CAD build for the part. Positions are in the model's coordinates, mm. Face numbers are marked on the shaded views. A direction names the side the tool comes from. Give positions to 0.01 mm unless a question says otherwise; leave off trailing zeros. Loops run counter-clockwise (first coordinate to the right, second up) from the corner with the lowest first, then second, coordinate; pieces in that order, holes last.
Autodesk Inventor part; units mm, degrees
ref_plane "YZ Plane" through (0, 0, 0) normal (1, 0, 0) x (0, 1, 0)
ref_plane "XZ Plane" through (0, 0, 0) normal (0, 1, 0) x (-1, 0, 0)
ref_plane "XY Plane" through (0, 0, 0) normal (0, 0, 1) x (1, 0, 0)
sketch "草图1" plane through (0, 0, 0) normal (0, 0, 1) x (1, 0, 0)
  circle A0 centre (0, 0) radius 4
  dimension "d0" = 8
extrude "拉伸1" add sketch "草图1" along normal blind 1
sketch "草图2" plane through (0, 0, 1) normal (0, 0, 1) x (1, 0, 0)
  line L0 (0, -2.8868) -> (-2.5, -1.4434)
  line L1 (-2.5, -1.4434) -> (-2.5, 1.4434)
  line L2 (-2.5, 1.4434) -> (0, 2.8868)
  line L3 (0, 2.8868) -> (2.5, 1.4434)
  line L4 (2.5, 1.4434) -> (2.5, -1.4434)
  line L5 (2.5, -1.4434) -> (0, -2.8868)
  point P0 (0, 0)
  point P1 (0, 0)
  dimension "d3" = 5
extrude "拉伸2" add sketch "草图2" along normal blind 4
sketch "草图3" plane through (0, 0, 0) normal (0, 0, -1) x (-1, 0, 0)
  circle A0 centre (0, 0) radius 2.5
  dimension "d6" = 5
extrude "拉伸3" add sketch "草图3" along normal blind 28
thread "螺纹1"
chamfer "倒角1" distance 0.25 angle 45 1 edges at (2.5, 0, -28)
properties part number "装填盘轴盖螺丝"
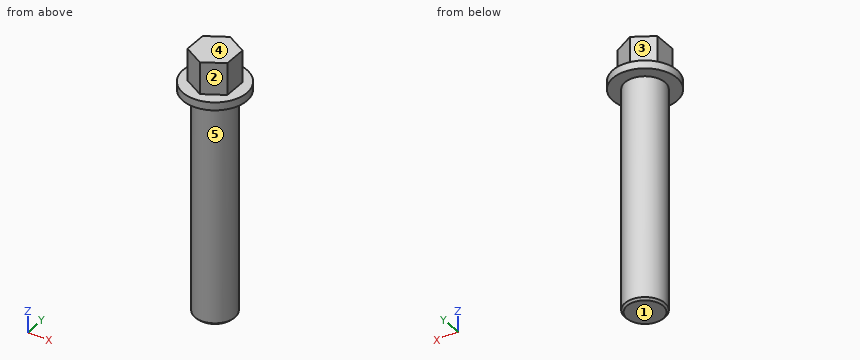
1. Saw through at D-D, the plane z = -8.5. List the corners of the cut face in (x, y), and give its area (3 significant figures).
Responses:
outline: circle Ø5 at (0, 0)
area: 19.6 mm2
2. Saw through at A-A, the plane y = 0. List the corners of the cut face in (x, z).
Responses:
outline: (-4, 0) - (-2.5, 0) - (-2.5, -27.75) - (-2.25, -28) - (2.25, -28) - (2.5, -27.75) - (2.5, 0) - (4, 0) - (4, 1) - (2.5, 1) - (2.5, 5) - (-2.5, 5) - (-2.5, 1) - (-4, 1) - close
3. Tool access for the marked faces 1, 2, 3, 4 and 5: list every direction of +Z, -Z, +X, -X, +Y, -Y with a clear straight run to the whole face (end or side of a thin tool).
Responses:
face 1: -Z, +X, -X, +Y, -Y
face 2: +Z, +X, -Y
face 3: +Z, -X, +Y
face 4: +Z, +X, -X, +Y, -Y
face 5: -Z
4. Probe line 1 along Z through (x, y) = (-0.5, -2.5); line 2 along Y through (x, z) = (0, -12); line 3 along Z through (x, y) = (-2.75, 0.5). List the from-to ranges inside material, lowest first.
Responses:
line 1: z = 0 to 5
line 2: y = -2.5 to 2.5
line 3: z = 0 to 1
5. Saw through at C-C, the plane x = 3. List the corners of the cut face in (y, z).
Responses:
outline: (-2.65, 0) - (2.65, 0) - (2.65, 1) - (-2.65, 1) - close
6. Saw through at B-B, the plane z = 1.5. List the corners of the cut face in (x, y).
Responses:
outline: (-2.5, -1.44) - (0, -2.89) - (2.5, -1.44) - (2.5, 1.44) - (0, 2.89) - (-2.5, 1.44) - close
7. Drop flat-ended pins along their axis: pin 1 (1.5 mm diameter, centred on y = -2.5, z = -13.5, fed in from +X); pin 2 (1.4 mm diameter, centred on y = 0.5, z = 3.5, fed in from +X); pin 3 (2.5 mm diameter, centred on y = -0.5, z = 3.5, fed in from -X). Give the stop position or say it passes through.
Responses:
pin 1: stops at x = 1.79
pin 2: stops at x = 2.5
pin 3: stops at x = -2.5
